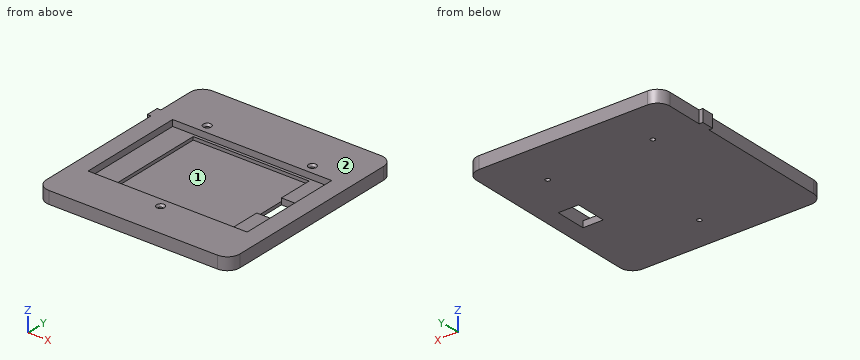
```python
from build123d import *

# Parameters (mm, degrees)
F2_R           = 1.85
F2_W           = 3
F2_H           = 10
F3_DEPTH       = 10
F4_DEPTH       = 5
F5_DEPTH       = 7.5
F6_D           = 3.7
F6_CSINK_D     = 6.4
F6_CSINK_ANGLE = 78


with BuildPart() as f3:
    # F2 (on offset) → F3 (new body)
    with BuildSketch(Plane.XY.offset(10)):
        with BuildLine():
            ThreePointArc((77.65, 72.65), (74.7210678119, 79.7210678119), (67.65, 82.65))
            Line((67.65, 82.65), (-67.65, 82.65))
            ThreePointArc((-67.65, 82.65), (-74.7210678119, 79.7210678119), (-77.65, 72.65))
            Line((-77.65, 72.65), (-77.65, 43.15))
            Line((-77.65, 43.15), (-77.65, 33.15))
            Line((-77.65, 33.15), (-77.65, -72.65))
            ThreePointArc((-77.65, -72.65), (-74.7210678119, -79.7210678119), (-67.65, -82.65))
            Line((-67.65, -82.65), (67.65, -82.65))
            ThreePointArc((67.65, -82.65), (74.7210678119, -79.7210678119), (77.65, -72.65))
            Line((77.65, -72.65), (77.65, 72.65))
        make_face()
        with Locations((0, -55)):
            Circle(F2_R, mode=Mode.SUBTRACT)
        Polygon((-64.15, -47.55), (-64.15, 37.95), (63.55, 37.95), (63.55, 7.7), (63.55, -17.3), (63.55, -47.55), align=None, mode=Mode.SUBTRACT)
        with Locations((-42.2, 45.3)):
            Circle(F2_R, mode=Mode.SUBTRACT)
        with Locations((42.2, 45.3)):
            Circle(F2_R, mode=Mode.SUBTRACT)
        Polygon((63.55, 37.95), (-64.15, 37.95), (-64.15, -47.55), (63.55, -47.55), (63.55, -17.3), (47.2, -17.3), (47.2, -45.3), (-45.8, -45.3), (-45.8, 35.7), (47.2, 35.7), (47.2, 7.7), (63.55, 7.7), align=None)
        with Locations((-79.15, 38.15)):
            Rectangle(F2_W, F2_H)
        Polygon((47.2, -17.3), (47.2, 7.7), (47.2, 35.7), (-45.8, 35.7), (-45.8, -45.3), (47.2, -45.3), align=None)
    extrude(amount=-F3_DEPTH)

    # F2 (on offset) → F4 (cut)
    with BuildSketch(Plane.XY.offset(10)):
        Polygon((63.55, 37.95), (-64.15, 37.95), (-64.15, -47.55), (63.55, -47.55), (63.55, -17.3), (47.2, -17.3), (47.2, -45.3), (-45.8, -45.3), (-45.8, 35.7), (47.2, 35.7), (47.2, 7.7), (63.55, 7.7), align=None)
    extrude(amount=-F4_DEPTH, mode=Mode.SUBTRACT)

    # F2 (on offset) → F5 (cut)
    with BuildSketch(Plane.XY.offset(10)):
        Polygon((47.2, -17.3), (47.2, 7.7), (47.2, 35.7), (-45.8, 35.7), (-45.8, -45.3), (47.2, -45.3), align=None)
    extrude(amount=-F5_DEPTH, mode=Mode.SUBTRACT)

    # F6 (through all)
    with Locations(Plane.XY.offset(10)):
        with Locations((-42.2, 45.3), (42.2, 45.3), (0, -55)):
            CounterSinkHole(F6_D / 2, F6_CSINK_D / 2, counter_sink_angle=F6_CSINK_ANGLE)


solid = f3.part
```
Could you check a few things on this model? Use its own coordinates, in mm. Face numbers are marked on the shaded views. A direction names the side the tool comes from. Coordinates: 2 decimals unless noted, no trailing zeros. Loops run counter-clockwise (first coordinate to the right, second up) from the corner with the lowest first, then second, coordinate; pieces in that order, holes last.
1) Imagine slicing it at C-C (y = 45.3). List the corners of the cut face in (x, z) for me.
Reported:
outline: (-77.65, 0) - (-44.05, 0) - (-44.05, 8.33) - (-45.4, 10) - (-77.65, 10) - close; (-40.35, 0) - (40.35, 0) - (40.35, 8.33) - (39, 10) - (-39, 10) - (-40.35, 8.33) - close; (44.05, 0) - (77.65, 0) - (77.65, 10) - (45.4, 10) - (44.05, 8.33) - close
2) Imagine slicing it at D-D (x = 6). List the corners of the cut face in (y, z) for me, and give its area (3 significant figures).
Reported:
outline: (-82.65, 0) - (82.65, 0) - (82.65, 10) - (37.95, 10) - (37.95, 5) - (35.7, 5) - (35.7, 2.5) - (-45.3, 2.5) - (-45.3, 5) - (-47.55, 5) - (-47.55, 10) - (-82.65, 10) - close
area: 1,020 mm2
3) Imagine slicing it at B-B (x = -42.2). List the corners of the cut face in (y, z) for me, and give its area (3 significant figures).
Reported:
outline: (-82.65, 0) - (43.45, 0) - (43.45, 8.33) - (42.1, 10) - (37.95, 10) - (37.95, 5) - (35.7, 5) - (35.7, 2.5) - (-45.3, 2.5) - (-45.3, 5) - (-47.55, 5) - (-47.55, 10) - (-82.65, 10) - close; (47.15, 0) - (82.65, 0) - (82.65, 10) - (48.5, 10) - (47.15, 8.33) - close
area: 984 mm2
4) Imagine slicing it at A-A (y = -55). List the corners of the cut face in (x, z) for me, and give its area (3 significant figures).
Reported:
outline: (-77.65, 0) - (-1.85, 0) - (-1.85, 8.33) - (-3.2, 10) - (-77.65, 10) - close; (1.85, 0) - (77.65, 0) - (77.65, 10) - (3.2, 10) - (1.85, 8.33) - close
area: 1,510 mm2
5) Will these pins go through, and if not, where does the flat tip stop? pin 1 Ø1.5 at (x, y) = (-53.5, -30.5) entering from +Z; pin 2 Ø1 at (x, y) = (39, -21) entering from +Z; pin 3 Ø3 at (y, z) = (50.5, 4) entering from -X.
Reported:
pin 1: stops at z = 5
pin 2: stops at z = 2.5
pin 3: stops at x = -77.65
6) Which directions (+Z, -Z, +X, -X, +Y, -Y) give clear straight access to the entire face, cutting with the end or side of a thin tool? Please do the marked faces 1 and 2.
Reported:
face 1: +Z
face 2: +Z, +X, -X, +Y, -Y
7) Please list where these lines run through material, in increasing order: line 1 along Y through (x, z) = (42.2, 5.25); line 2 along X through (y, z) = (45.3, 6.5); line 3 along Y through (x, z) = (42.2, 3.5).
Reported:
line 1: y = -82.65 to -47.55, 37.95 to 43.45, 47.15 to 82.65
line 2: x = -77.65 to -44.05, -40.35 to 40.35, 44.05 to 77.65
line 3: y = -82.65 to -45.3, 35.7 to 43.45, 47.15 to 82.65
